```python
from build123d import *

# Parameters (mm, degrees)
SKETCH_1_R      = 73
SKETCH_1_R_2    = 71.5
EXTRUDE_1_DEPTH = 11
SKETCH_2_R      = 71.5
SKETCH_2_R_2    = 61
EXTRUDE_2_DEPTH = 3
SKETCH_3_R      = 61
SKETCH_3_R_2    = 59.5
EXTRUDE_3_DEPTH = 10
EXTRUDE_START   = 7
SKETCH_4_R      = 59.5
EXTRUDE_4_DEPTH = 3
EXTRUDE_5_DEPTH = 7


with BuildPart() as part:
    # 스케치1 → 보스-돌출1 (new body)
    with BuildSketch(Plane(origin=(0, 0, 0), x_dir=(1, 0, 0), z_dir=(0, 1, 0))):
        with Locations(Location((0, 0, 0), (0, 0, 270))):
            Circle(SKETCH_1_R)
        with Locations(Location((0, 0, 0), (0, 0, 270))):
            Circle(SKETCH_1_R_2, mode=Mode.SUBTRACT)
    extrude(amount=EXTRUDE_1_DEPTH)

    # 스케치2 → 보스-돌출2 (add)
    with BuildSketch(Plane(origin=(0, 0, 0), x_dir=(1, 0, 0), z_dir=(0, 1, 0))):
        with Locations(Location((0, 0, 0), (0, 0, 270))):
            Circle(SKETCH_2_R)
        with Locations(Location((0, 0, 0), (0, 0, 270))):
            Circle(SKETCH_2_R_2, mode=Mode.SUBTRACT)
    extrude(amount=EXTRUDE_2_DEPTH)

    # 스케치3 → 보스-돌출3 (add)
    with BuildSketch(Plane(origin=(0, 0, 0), x_dir=(1, 0, 0), z_dir=(0, 1, 0))):
        with Locations(Location((0, 0, 0), (0, 0, 270))):
            Circle(SKETCH_3_R)
        with Locations(Location((0, 0, 0), (0, 0, 270))):
            Circle(SKETCH_3_R_2, mode=Mode.SUBTRACT)
    extrude(amount=EXTRUDE_3_DEPTH)

    # 스케치4 → 보스-돌출4 (add)
    with BuildSketch(Plane(origin=(0, 0, 0), x_dir=(1, 0, 0), z_dir=(0, 1, 0)).offset(EXTRUDE_START)):
        with Locations(Location((0, 0, 0), (0, 0, 270))):
            Circle(SKETCH_4_R)
    extrude(amount=EXTRUDE_4_DEPTH)

    # 스케치6 → 보스-돌출5 (add)
    with BuildSketch(Plane.XZ.offset(-7).offset(EXTRUDE_START)):
        with BuildLine():
            Line((-1.804298071, 9.835878632), (-10.73557352, 58.523477863))
            ThreePointArc((-10.73557352, 58.523477863), (-8.172597382, 58.93605562), (-5.594064241, 59.236445245))
            Line((-5.594064241, 59.236445245), (-0.940178864, 9.955705083))
            ThreePointArc((-0.940178864, 9.955705083), (7.891398769, 6.142135253), (9.4202698, -3.355371351))
            Line((9.4202698, -3.355371351), (56.050605307, -19.964459539))
            ThreePointArc((56.050605307, -19.964459539), (55.126420057, -22.390350862), (54.097298532, -24.77362088))
            Line((54.097298532, -24.77362088), (9.091982947, -4.163633761))
            ThreePointArc((9.091982947, -4.163633761), (1.373545779, -9.905219432), (-7.615971729, -6.480507281))
            Line((-7.615971729, -6.480507281), (-45.315031787, -38.559018324))
            ThreePointArc((-45.315031787, -38.559018324), (-46.953822675, -36.545704758), (-48.503234292, -34.462824365))
            Line((-48.503234292, -34.462824365), (-8.151804083, -5.792071322))
            ThreePointArc((-8.151804083, -5.792071322), (-9.264944547, 3.763084178), (-1.804298071, 9.835878632))
        make_face()
    extrude(amount=-EXTRUDE_5_DEPTH)


solid = part.part
```
Build history of the part. All positions in model axes, mm. A direction names the side the tool comes from. Coordinates: 2 decimals unless noted, no trailing zeros. Order: outer loops, then holes, each group sorted by start corner. A loop starts at its lowest first (then second) coordinate and runs counter-clockwise, first axis right, second up. Notation, with made-up numbers: M -20.75,67.25 L 31.25,67.25 A22 ccw 31.25,73.25 Z; hole C 23.5,17.5 d4. An arc over 180 degrees is marked long. One line per question, with ' | ' between items. Start each with the question number.
1. Wall check: line 1 along X through (y, z) = (5, 0); line 2 along X through (y, z) = (8, 0); line 3 along X through (y, z) = (6.5, -50.5). Give the ranges that are in metal, low to high. Write a range as [from, to].
2. Flat gauge pins, fed straight in: P1, Ø1.5, axis at x = 3, y = 7, coming from the -Z side; P2, Ø2, axis at x = 13.5, z = 57, coming from the +Y side; P3, Ø1.5, axis at y = 6, z = 32.5, coming from the +X side. Where does each tip first touch, or does it go through?
3. Tool access for faces 3 (the face through (-59.55, 6.45, -13.22)), 4 (the face through (9, 3.451, -58.815)), 5 (the face through (-54, 11, 48)): list every direction of +Z, -Z, +X, -X, +Y, -Y with a clear straight run to the whole face (end or side of a thin tool).
4. Cut at C-C (z = -36.5). Write the cut outline in (x, y).
5. Cut at A-A (z = 0). Write the cut outline in (x, y).
6. Mould opens along X. For faces 1 (the face through (-9.32, 3.45, 3.63)), 2 (the face through (0, 0, -6)) say: +X half, -X half, draft (parallel to the pull), parting line (faces both ways), or undercut.
7. Cut at B-B (x = -29). Write the cut outline in (y, z), plus the area to 3 significant figures.
The answers:
1) line 1: x = [-73, -71.5], [-61, -59.5], [-10, 10], [59.5, 61], [71.5, 73] | line 2: x = [-73, -71.5], [-61, 61], [71.5, 73] | line 3: x = [-52.71, -50.62], [-34.22, -31.46], [31.46, 34.22], [50.62, 52.71]
2) P1: stops at z = -72.97 | P2: stops at y = 10 | P3: stops at x = 65.73
3) face 3: +Y | face 4: -Y | face 5: +Z, -Z, +X, -X, +Y
4) outline: M -63.22,0 L -42.9,0 L -42.9,7 L 46.99,7 L 46.99,0 L 63.22,0 L 63.22,11 L 61.48,11 L 61.48,3 L 48.87,3 L 48.87,10 L -48.87,10 L -48.87,3 L -61.48,3 L -61.48,11 L -63.22,11 Z
5) outline: M -73,0 L -59.5,0 L -59.5,7 L -10,7 L -10,0 L 10,0 L 10,7 L 59.5,7 L 59.5,0 L 73,0 L 73,11 L 71.5,11 L 71.5,3 L 61,3 L 61,10 L -61,10 L -61,3 L -71.5,3 L -71.5,11 L -73,11 Z
6) face 1: undercut | face 2: draft
7) outline: M 0,-66.99 L 11,-66.99 L 11,-65.35 L 3,-65.35 L 3,-53.67 L 10,-53.67 L 10,53.67 L 3,53.67 L 3,65.35 L 11,65.35 L 11,66.99 L 0,66.99 L 0,51.95 L 7,51.95 L 7,-20.61 L 0,-20.61 L 0,-24.68 L 7,-24.68 L 7,-51.95 L 0,-51.95 Z | area: 481 mm2
